Could you check a few things on this model? Use its own coordinates, in mm. A direction names the side the tool comes from. Round coordinates to 2 decimals unless told otherwise and drop trailing zeros. Loops run counter-clockwise (first coordinate to the right, second up) from the corner with the lowest first, then second, coordinate; pieces in that order, holes last. Notation, with made-up numbers: (17, -16.75) -> (70, -16.75) arc R19 cw to (70, 10.25) -> close; hole circle Ø2 at (70, -12). An arc over 180 degrees is marked (long way). Use CSV: the item, a comma, the result in double quotes. Start each with the question number.
```python
from build123d import *

# Parameters (mm, degrees)
BOSS_EXTRUDE1_START = 22
BOSS_EXTRUDE1_DEPTH = 199


with BuildPart() as part:
    # Sketch1 → Boss-Extrude1 (new body)
    with BuildSketch(Plane.XY.offset(BOSS_EXTRUDE1_START)):
        Polygon((-22, 30), (-22, -114.5), (167.5, -183.472359393), (165.789899283, -188.170822497), (-27, -118.001037691), (-27, 30), align=None)
    extrude(amount=-BOSS_EXTRUDE1_DEPTH)


solid = part.part
```
1. If I drill on L1, parallel to X at y = -61.5, z = -27.5; L2, parallel to Y at x = 134.5, z = 12; L3, parallel to Y at x = 65, z = -16, over which ranges is the centre line in solid material (lowest first)?
2. Suppose I cut it at B-B (y = -104.5). List the corners of the cut face in (x, z) for me.
3. For faces 1 (the face through (-27, -45, -76)), 2 (the face through (-22, -41, -76)), which set-ups out of +Z, -Z, +X, -X, +Y, -Y let a thin tool reach every point of the face, with its end or its side?
4. Suppose I cut it at A-A (z = -81). List the corners of the cut face in (x, y) for me, then the cut area to 3 significant figures.
5. Will these pins go through, and if not, where does the flat tip stop? pin 1 (12 mm diameter, centred on x = 3, z = -135.5, fed in from -Y); pin 2 (5 mm diameter, centred on x = 49, z = -42.5, fed in from +Y); pin 3 (5 mm diameter, centred on y = -56, z = -144, fed in from +X).
6. Suppose I cut it at C-C (x = 70.5). List the corners of the cut face in (y, z) for me.
Geometry check:
1,L1,"x = -27 to -22"
1,L2,"y = -176.78 to -171.46"
1,L3,"y = -151.49 to -146.17"
2,outline,"(-27, -177) -> (-22, -177) -> (-22, 22) -> (-27, 22) -> close"
3,face 1,"+Z, -Z, -X, +Y, -Y"
3,face 2,"+Z, -Z, +X, +Y"
4,outline,"(-27, -118) -> (165.79, -188.17) -> (167.5, -183.47) -> (-22, -114.5) -> (-22, 30) -> (-27, 30) -> close"
4,area,"1,750 mm²"
5,pin 1,"stops at y = -131.1"
5,pin 2,"stops at y = -139.43"
5,pin 3,"stops at x = -22"
6,outline,"(-153.49, -177) -> (-148.17, -177) -> (-148.17, 22) -> (-153.49, 22) -> close"
